Could you check a few things on this model? Use its own coordinates, in mm. A direction names the side the tool comes from. Give positions to 0.01 mm unless a question says otherwise; leave off trailing zeros. Order: outer loops, then holes, each group sorted by start corner. A loop starts at its lowest first (then second) coordinate and runs counter-clockwise, first axis right, second up.
(1) Imagine slicing it at D-D, the plane z = -40.5. Write out the boundary of the cut face in (x, y), then the cut area to 3 significant figures.
(2) On a 3-axis mill with a long thin cutter (end or side, diameter ignored), from which of +Z, -Z, +X, -X, +Y, -Y can I reach the whole of each face in a straight line? I mean faces 1 (the flat face through (5, 2, -5)), 2 (the flat face through (0, 7, -49)), 3 (the flat face through (49, 10, 13)), 4 (the flat face through (50, 15, 0)), 5 (the flat face through (15, 10, -50)). Say none if no direction works.
(3) Imagine slicing it at C-C, the plane x = 58.5. Write out the boundary of the cut face in (y, z).
(4) Imagine slicing it at B-B, the plane y = 10. State how many separate pieces and enclosed holes the cut face has, then the cut area to 3 significant figures.
(5) Will these pins go through, and if not, where does the flat tip stop? pin 1 (1 mm diameter, centred on y = 11.5, z = -17.5, fed in from +X); pin 2 (6.5 mm diameter, centred on y = 11.5, z = -54, fed in from +X); pin 3 (2 mm diameter, centred on x = 45.5, y = 2.5, fed in from +Z); pin 4 (11 mm diameter, centred on x = 59.5, y = 8.5, fed in from +Z).
(6) If I drill on probe 1 along Z at (x, y) = (50, 8); probe 2 along Y at (x, z) = (15, 9.5); probe 3 along X at (y, z) = (4.5, -9), over which ranges is the centre line in solid material (lowest first)?
(7) If we mould it in two halves opening along Z, with no side actions, what happens to faces 6 (the flat face through (30, 17, 0)), 7 (the flat face through (49, 7, 0)), 8 (the flat face through (50, 10, 15))? For each: released by +Z, released by -Z, zero draft, split by the parting line, or undercut.
(8) Imagine slicing it at A-A, the plane z = -5. Write out the boundary of the cut face in (x, y), then the cut area to 3 significant figures.
from build123d import *

# Parameters (mm, degrees)
CROQUIS1_W     = 40
CROQUIS1_H     = 50
CROQUIS1_H_2   = 40
CROQUIS1_W_2   = 50
EXTRUIR1_DEPTH = 20
CROQUIS2_W     = 40
CROQUIS2_H     = 20
CROQUIS2_W_2   = 30
CROQUIS2_H_2   = 10
EXTRUIR2_DEPTH = 40
CROQUIS3_W     = 40
CROQUIS3_H     = 20
CROQUIS3_W_2   = 30
CROQUIS3_H_2   = 10
EXTRUIR3_DEPTH = 40
VACIADO1_T     = -2
CROQUIS5_R     = 5
EXTRUIR4_DEPTH = 10


with BuildPart() as part:
    # Croquis1 → Extruir1 (new body)
    with BuildSketch(Plane(origin=(0, 0, 0), x_dir=(1, 0, 0), z_dir=(0, 1, 0))):
        with Locations((0, 45)):
            Rectangle(CROQUIS1_W, CROQUIS1_H)
        Rectangle(CROQUIS1_W, CROQUIS1_H_2)
        with Locations((45, 0)):
            Rectangle(CROQUIS1_W_2, CROQUIS1_H_2)
    extrude(amount=EXTRUIR1_DEPTH)

    # Croquis2 → Extruir2 (cut)
    with BuildSketch(Plane(origin=(70, 0, 0), x_dir=(0, 0, -1), z_dir=(1, 0, 0))):
        with Locations((0, 10)):
            Rectangle(CROQUIS2_W, CROQUIS2_H)
        with Locations((0, 10)):
            Rectangle(CROQUIS2_W_2, CROQUIS2_H_2, mode=Mode.SUBTRACT)
    extrude(amount=-EXTRUIR2_DEPTH, mode=Mode.SUBTRACT)

    # Croquis3 → Extruir3 (cut)
    with BuildSketch(Plane(origin=(0, 0, -70), x_dir=(-1, 0, 0), z_dir=(0, 0, -1))):
        with Locations((0, 10)):
            Rectangle(CROQUIS3_W, CROQUIS3_H)
        with Locations((0, 10)):
            Rectangle(CROQUIS3_W_2, CROQUIS3_H_2, mode=Mode.SUBTRACT)
    extrude(amount=-EXTRUIR3_DEPTH, mode=Mode.SUBTRACT)

    # Vaciado1
    vaciado1_openings = [part.faces().sort_by_distance(p)[0] for p in [
        (70, 10, 0),
        (0, 10, -70),
    ]]
    offset(amount=VACIADO1_T, openings=vaciado1_openings, kind=Kind.INTERSECTION)

    # Croquis5 → Extruir4 (cut)
    with BuildSketch(Plane.ZY.offset(20)):
        with Locations((-5, 10)):
            Circle(CROQUIS5_R)
    extrude(amount=-EXTRUIR4_DEPTH, mode=Mode.SUBTRACT)


solid = part.part
Answer block:
1. outline: (-15, 5) - (15, 5) - (15, 15) - (-15, 15) - close; hole (-13, 7) - (13, 7) - (13, 13) - (-13, 13) - close
1. area: 144 mm2
2. face 1: none
2. face 2: -Z
2. face 3: +X
2. face 4: +Z, -Z, +X, +Y
2. face 5: -Z, +X, +Y, -Y
3. outline: (5, -15) - (15, -15) - (15, 15) - (5, 15) - close; hole (7, -13) - (13, -13) - (13, 13) - (7, 13) - close
4. separate pieces: 3
4. enclosed holes: 0
4. area: 580 mm2
5. pin 1: stops at x = 30
5. pin 2: stops at x = 15
5. pin 3: passes through
5. pin 4: stops at z = 15
6. probe 1: z = -15 to -13, 13 to 15
6. probe 2: y = 0 to 2, 18 to 20
6. probe 3: x = -20 to -18, 28 to 30
7. face 6: zero draft
7. face 7: undercut
7. face 8: released by +Z
8. outline: (-20, 0) - (30, 0) - (30, 5) - (70, 5) - (70, 7) - (28, 7) - (28, 2) - (-18, 2) - (-18, 5) - (-20, 5) - close; (-20, 15) - (-18, 15) - (-18, 18) - (28, 18) - (28, 13) - (70, 13) - (70, 15) - (30, 15) - (30, 20) - (-20, 20) - close
8. area: 392 mm2
